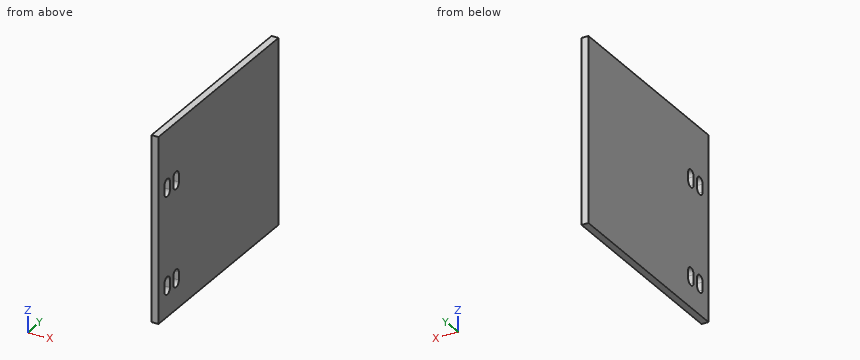
Autodesk Inventor part; units mm, degrees
ref_plane "YZ Plane" through (0, 0, 0) normal (1, 0, 0) x (0, 1, 0)
ref_plane "XZ Plane" through (0, 0, 0) normal (0, 1, 0) x (-1, 0, 0)
ref_plane "XY Plane" through (0, 0, 0) normal (0, 0, 1) x (1, 0, 0)
sketch "Sketch1" plane through (0, 0, 0) normal (0, 0, 1) x (1, 0, 0)
  point P0 (0, 0)
sketch "Sketch2" plane through (0, 0, 0) normal (1, 0, 0) x (0, 1, 0)
  line L0 (0, 0) -> (-152.4, 0)
  line L1 (-152.4, 0) -> (-152.4, -133.35)
  line L2 (-152.4, -133.35) -> (0, -133.35)
  line L3 (0, -133.35) -> (0, 0)
  dimension "d0" = 152.4
  dimension "d1" = 133.35
extrude "Extrusion1" add sketch "Sketch2" along normal blind 5.08
sketch "Sketch6" plane through (5.08, 0, 0) normal (1, 0, 0) x (0, 0, -1)
  line L0 (0, -152.4) -> (133.35, -152.4)
  line L1 (133.35, -152.4) -> (133.35, 0)
  line L2 (0, 0) -> (0, -152.4)
  line L3 (41.275, -130.048) -> (47.625, -130.048)
  line L4 (47.625, -130.048) -> (41.275, -130.048)
  line L5 (41.275, -130.048) -> (34.925, -130.048)
  line L6 (34.925, -130.048) -> (47.625, -130.048) construction
  line L7 (38.4175, -133.5405) -> (44.1325, -133.5405)
  line L8 (44.1325, -126.5555) -> (38.4175, -126.5555)
  arc A0 (38.4175, -126.5555) -> (38.4175, -133.5405) centre (38.4175, -130.048) ccw
  arc A1 (44.1325, -133.5405) -> (44.1325, -126.5555) centre (44.1325, -130.048) ccw
  line L9 (111.125, -130.048) -> (117.475, -130.048)
  line L10 (117.475, -130.048) -> (111.125, -130.048)
  line L11 (111.125, -130.048) -> (104.775, -130.048)
  line L12 (104.775, -130.048) -> (117.475, -130.048) construction
  line L13 (108.2675, -133.5405) -> (113.9825, -133.5405)
  line L14 (113.9825, -126.5555) -> (108.2675, -126.5555)
  arc A2 (108.2675, -126.5555) -> (108.2675, -133.5405) centre (108.2675, -130.048) ccw
  arc A3 (113.9825, -133.5405) -> (113.9825, -126.5555) centre (113.9825, -130.048) ccw
  line L15 (41.275, -141.351) -> (47.625, -141.351)
  line L16 (47.625, -141.351) -> (41.275, -141.351)
  line L17 (41.275, -141.351) -> (34.925, -141.351)
  line L18 (34.925, -141.351) -> (47.625, -141.351) construction
  line L19 (38.4175, -144.8435) -> (44.1325, -144.8435)
  line L20 (44.1325, -137.8585) -> (38.4175, -137.8585)
  arc A4 (38.4175, -137.8585) -> (38.4175, -144.8435) centre (38.4175, -141.351) ccw
  arc A5 (44.1325, -144.8435) -> (44.1325, -137.8585) centre (44.1325, -141.351) ccw
  line L21 (111.125, -141.351) -> (117.475, -141.351)
  line L22 (111.125, -141.351) -> (104.775, -141.351)
  line L23 (104.775, -141.351) -> (117.475, -141.351) construction
  line L24 (108.2675, -144.8435) -> (113.9825, -144.8435)
  line L25 (113.9825, -137.8585) -> (108.2675, -137.8585)
  arc A6 (108.2675, -137.8585) -> (108.2675, -144.8435) centre (108.2675, -141.351) ccw
  arc A7 (113.9825, -144.8435) -> (113.9825, -137.8585) centre (113.9825, -141.351) ccw
  dimension "d28" = 6.35
  dimension "d30" = 6.985
  dimension "d31" = 6.35
  dimension "d32" = 6.35
  dimension "d33" = 6.985
  dimension "d34" = 6.35
  dimension "d35" = 6.35
  dimension "d36" = 6.985
  dimension "d37" = 6.35
  dimension "d38" = 6.35
  dimension "d39" = 6.985
extrude "Extrusion5" cut sketch "Sketch6" against normal blind 25.4
properties part number "HalfFrontWall"
Could you check a few things on this model? Use its own coordinates, in mm. Round coordinates to 2 decimals unless told otherwise and drop trailing zeros. Put each result on its own line as item: value. Start each with the question number.
(1) I need wall thicknesses on probe 1 along Y at (x, z) = (0.2, -113); probe 2 along Y at (x, z) = (3.6, -107). Which ranges of each line are inside material? Lowest first, please.
(2) I want a section at A-A, the plane x = 3.6. Give the number of separate pieces and of enclosed holes in the cut face, plus the area to 3 significant figures.
(3) Will this pin go through, and if not, where does the flat tip stop? pin 1 (3 mm diameter, centred on x = 1, z = -119, fed in from +Y).
Here are the results:
1. probe 1: y = -152.4 to -144.84, -137.86 to -133.54, -126.56 to 0
1. probe 2: y = -152.4 to -144.61, -138.1 to -133.3, -126.79 to 0
2. separate pieces: 1
2. enclosed holes: 4
2. area: 20,000 mm^2
3. pin 1: stops at y = 0
